```python
from build123d import *

# Parameters (mm, degrees)
ESQUISSE2_W                  = 6
ESQUISSE2_H                  = 6
ESQUISSE3_R                  = 50
BOSS_EXTRU_1_DEPTH           = 3
R_P_TITION_CIRCULAIRE1_COUNT = 3


with BuildPart() as part:
    # Balayage2: sweep along a curve in space
    with BuildLine() as balayage2_path:
        Line((0, 0, 0), (0, 0, -176.45))
        Line((0, 0, -176.45), (0, 550, -176.45))
    # Esquisse2 → Balayage2 (sweep)
    with BuildSketch(Plane.XY):
        Rectangle(ESQUISSE2_W, ESQUISSE2_H)
    balayage2 = sweep(path=balayage2_path.line, transition=Transition.RIGHT)

    # Esquisse3 → Boss.-Extru.1 (add, symmetric)
    with BuildSketch(Plane(origin=(0, 0, 0), x_dir=(1, 0, 0), z_dir=(0, 1, 0))):
        Circle(ESQUISSE3_R)
    extrude(amount=BOSS_EXTRU_1_DEPTH, both=True)

    # Répétition circulaire1: Balayage2 ×3 about axis
    r_p_tition_circulaire1_axis = Axis((0, 0, 0), (0, 1, 0))
    for i in range(1, R_P_TITION_CIRCULAIRE1_COUNT):
        add(balayage2.rotate(r_p_tition_circulaire1_axis, i * 360 / R_P_TITION_CIRCULAIRE1_COUNT))


solid = part.part
```
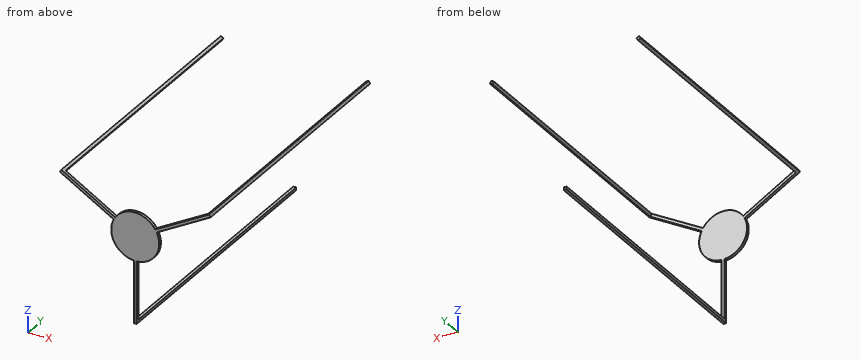
Check sheet for the modelled part. Datum: model origin and axes. Units: mm. Give positions to 0.01 mm unless a question says otherwise; leave off trailing zeros. Order: outer loops, then holes, each group sorted by start corner. A loop starts at its lowest first (then second) coordinate and runs counter-clockwise, first axis right, second up. Notation, with made-up numbers: (-38, -30.75) -> (-30, -30.75) arc R11 cw to (-30, -11.75) -> close; hole circle Ø2 at (1, 67.25). An arc over 180 degrees is marked (long way). Use CSV: the item, a comma, the result in double quotes. Start each with the question number.
1) Sectioned sample at D-D, the plane x = 16. Record the boundary of the cut face in (y, z), plus the area to 3 significant figures.
2) Go/stop test with a flat-tipped pin: P1, Ø6.5, axis at x = 1, y = 404.5, coming from the +Z side. Record where the tip stops, or that it passes through.
3) Material ranges on line 1 (Y direction, x = -12.5, z = 4); line 2 (Z direction, x = 0, y = 394), recorded low to high. Write a range as from..to.
4) Sectioned sample at B-B, the plane z = 66. Record the boundary of the cut face in (x, y).
5) Sectioned sample at C-C, the plane z = -130. Record the boundary of the cut face in (x, y), plus the area to 3 significant figures.
6) Sectioned sample at A-A, the plane y = 127. Record the boundary of the cut face in (x, z).
Recorded:
1,outline,"(-3, -47.37) -> (3, -47.37) -> (3, 47.37) -> (-3, 47.37) -> close"
1,area,"568 mm2"
2,P1,"z = -173.45"
3,line 1,"-3..3"
3,line 2,"-179.45..-173.45"
4,outline,"(-120.32, -3) -> (-108.32, -3) -> (-108.32, 3) -> (-120.32, 3) -> close; (108.32, -3) -> (120.32, -3) -> (120.32, 3) -> (108.32, 3) -> close"
5,outline,"(-3, -3) -> (3, -3) -> (3, 3) -> (-3, 3) -> close"
5,area,"36.0 mm2"
6,outline,"(-156.91, 87.13) -> (-151.71, 84.13) -> (-148.71, 89.32) -> (-153.91, 92.32) -> close; (-3, -179.45) -> (3, -179.45) -> (3, -173.45) -> (-3, -173.45) -> close; (148.71, 89.32) -> (151.71, 84.13) -> (156.91, 87.13) -> (153.91, 92.32) -> close"
